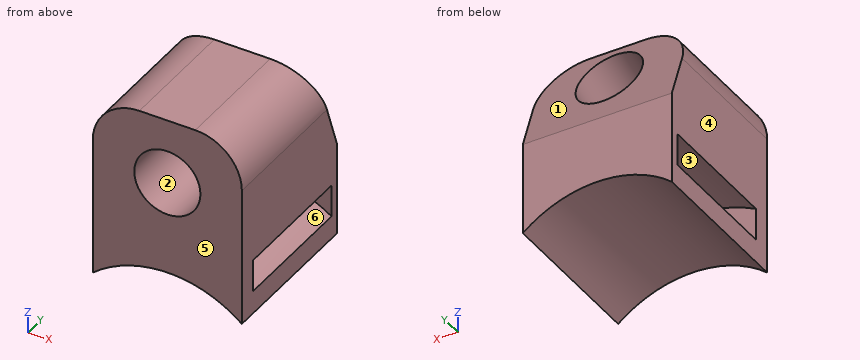
```python
from build123d import *

# Parameters (mm, degrees)
F1_DEPTH  = 15
F3_DEPTH  = 2
F5_R      = 3.55
F8_DEPTH  = 25
F11_DEPTH = 1
F12_R     = 5


with BuildPart() as f1:
    # F0 (on Front) → F1 (new body)
    with BuildSketch(Plane.XZ):
        with BuildLine():
            ThreePointArc((-8, 9.6046863561), (0, 12.5), (8, 9.6046863561))
            Line((8, 9.6046863561), (8, 12.0933866224))
            ThreePointArc((8, 12.0933866224), (0, 14.5), (-8, 12.0933866224))
            Line((-8, 12.0933866224), (-8, 9.6046863561))
        make_face()
    extrude(amount=F1_DEPTH)


with BuildPart() as f1b:
    # F0 (on Front) → F1, piece 2 (new body)
    with BuildSketch(Plane.XZ):
        with BuildLine():
            ThreePointArc((-8, 15.5643824163), (0, 17.5), (8, 15.5643824163))
            Line((8, 15.5643824163), (8, 29.5643824163))
            Line((8, 29.5643824163), (-8, 29.5643824163))
            Line((-8, 29.5643824163), (-8, 15.5643824163))
        make_face()
    extrude(amount=F1_DEPTH)


with BuildPart() as f3:
    # F2 (on face) → F3 (new body)
    with BuildSketch(Plane.XZ.offset(15)):
        with BuildLine():
            ThreePointArc((-8, 9.6046863561), (0, 12.5), (8, 9.6046863561))
            Line((8, 9.6046863561), (8, 12.0933866224))
            ThreePointArc((8, 12.0933866224), (0, 14.5), (-8, 12.0933866224))
            Line((-8, 12.0933866224), (-8, 9.6046863561))
        make_face()
        with BuildLine():
            ThreePointArc((-8, 12.0933866224), (0, 14.5), (8, 12.0933866224))
            Line((8, 12.0933866224), (8, 15.5643824163))
            ThreePointArc((8, 15.5643824163), (0, 17.5), (-8, 15.5643824163))
            Line((-8, 15.5643824163), (-8, 12.0933866224))
        make_face()
        with BuildLine():
            ThreePointArc((-8, 15.5643824163), (0, 17.5), (8, 15.5643824163))
            Line((8, 15.5643824163), (8, 29.5643824163))
            Line((8, 29.5643824163), (-8, 29.5643824163))
            Line((-8, 29.5643824163), (-8, 15.5643824163))
        make_face()
    extrude(amount=F3_DEPTH)


with BuildPart() as f6_tool:
    # F6: sweep along a path in F4
    with BuildLine(Plane.YZ.offset(8)) as f6_path:
        Line((-16, 22.5643824163), (-10, 22.5643824163))
        Line((-10, 22.5643824163), (0, 26.2040847589))
        Line((0, 26.2040847589), (4.1724268391, 27.722723933))
    # F5 (on face) → F6 (sweep)
    with BuildSketch(Plane.XZ.offset(17)):
        with Locations((0, 22.5643824163)):
            Circle(F5_R)
    sweep(path=f6_path.line, transition=Transition.RIGHT)


with BuildPart() as f1b_1:
    add(f1b.part)

    # F6: cut by f6_tool
    add(f6_tool.part, mode=Mode.SUBTRACT)

    # F7 (on face) → F8 (cut)
    with BuildSketch(Plane.YZ.offset(8)):
        Polygon((-3.6397023427, 29.5643824163), (0, 19.5643824163), (0, 29.5643824163), align=None)
    extrude(amount=-F8_DEPTH, mode=Mode.SUBTRACT)


with BuildPart() as f3_1:
    add(f3.part)

    # F6: cut by f6_tool
    add(f6_tool.part, mode=Mode.SUBTRACT)


with BuildPart() as f1_1:
    add(f1.part)

    # F9: union F1b, F3
    add(f1b_1.part)
    add(f3_1.part)

    # F10 (on face) → F11 (join)
    with BuildSketch(Plane(origin=(0, 0, 0), x_dir=(-1, 0, 0), z_dir=(0, 1, 0))):
        with BuildLine():
            ThreePointArc((8, 12.0933866224), (0, 14.5), (-8, 12.0933866224))
            Line((-8, 12.0933866224), (-8, 9.6046863561))
            ThreePointArc((-8, 9.6046863561), (0, 12.5), (8, 9.6046863561))
            Line((8, 9.6046863561), (8, 12.0933866224))
        make_face()
        with BuildLine():
            Line((-8, 15.5643824163), (-8, 12.0933866224))
            ThreePointArc((-8, 12.0933866224), (0, 14.5), (8, 12.0933866224))
            Line((8, 12.0933866224), (8, 15.5643824163))
            ThreePointArc((8, 15.5643824163), (0, 17.5), (-8, 15.5643824163))
        make_face()
        with BuildLine():
            Line((-8, 19.5643824163), (-8, 15.5643824163))
            ThreePointArc((-8, 15.5643824163), (0, 17.5), (8, 15.5643824163))
            Line((8, 15.5643824163), (8, 19.5643824163))
            Line((8, 19.5643824163), (-8, 19.5643824163))
        make_face()
    extrude(amount=-F11_DEPTH)

    # F12
    f12_edges = [f1_1.edges().sort_by_distance(p)[0] for p in [
        (8, -10.319851, 29.564382),
        (-8, -10.319851, 29.564382),
    ]]
    fillet(f12_edges, radius=F12_R)


solid = f1_1.part
```
Part model, mm, in its own coordinate system. Face numbers are marked on the shaded views. A direction names the side the tool comes from. Round coordinates to 2 decimals unless told otherwise and drop trailing zeros. Loops run counter-clockwise (first coordinate to the right, second up) from the corner with the lowest first, then second, coordinate; pieces in that order, holes last. Notation, with made-up numbers: (-7.75, 68.25) -> (5.25, 68.25) arc R17 ccw to (5.25, 100.25) -> close; hole circle Ø5 at (3, 11). An arc over 180 degrees is marked (long way). Use a Markdown table: item, result.
1) Cut at A-A, the plane x = 0. List the corners of the cut face in (y, z), and give its area (3 significant figures).
The answers:
| item | result |
|---|---|
| outline | (-17, 12.5) -> (0, 12.5) -> (0, 19.56) -> (-0.92, 22.09) -> (-9.37, 19.01) -> (-17, 19.01) -> close; (-17, 26.11) -> (-10.63, 26.11) -> (-3.35, 28.76) -> (-3.64, 29.56) -> (-17, 29.56) -> close; hole (-15, 14.5) -> (-1, 14.5) -> (-1, 17.5) -> (-15, 17.5) -> close |
| area | 121 mm2 |
2) Drop a flat-ended pin along its axis: pin 1 Ø3 at (x, y) = (0, -3.5) entering from -Z. Give the stop position or say it passes through.
The answers:
| item | result |
|---|---|
| pin 1 | stops at z = 12.41 |
3) Pull direction Y, two halves, no side cores. Call the marked faces 4, 5 and 6: pulls with the +Y half, pulls with the -Y half, needs draft (parallel to the pull), parting line crosses it, or undercut.
The answers:
| item | result |
|---|---|
| face 4 | needs draft |
| face 5 | pulls with the -Y half |
| face 6 | undercut |
4) Tool access for the marked faces 1, 2 and 3: list every direction of +Z, -Z, +X, -X, +Y, -Y with a clear straight run to the whole face (end or side of a thin tool).
The answers:
| item | result |
|---|---|
| face 1 | +Z, +X, -X, +Y |
| face 2 | -Y |
| face 3 | none |
5) Probe line 1 (Z direction, x = 0, y = -14); line 2 (Y direction, x = 6.25, z = 14.5); line 3 (Z direction, x = 0, y = -15.25). List the from-to ranges inside material, lowest first. Write a range as [from, to].
The answers:
| item | result |
|---|---|
| line 1 | z = [12.5, 14.5], [17.5, 19.01], [26.11, 29.56] |
| line 2 | y = [-17, -15], [-1, 0] |
| line 3 | z = [12.5, 19.01], [26.11, 29.56] |
6) Cut at C-C, the plane z = 12.75. List the corners of the cut face in (x, y).
The answers:
| item | result |
|---|---|
| outline | (-8, -17) -> (8, -17) -> (8, -15) -> (6.91, -15) -> (6.91, -1) -> (8, -1) -> (8, 0) -> (-8, 0) -> (-8, -1) -> (-6.91, -1) -> (-6.91, -15) -> (-8, -15) -> close |
7) Cut at D-D, the plane x = 2.25. List the corners of the cut face in (y, z).
The answers:
| item | result |
|---|---|
| outline | (-17, 12.3) -> (0, 12.3) -> (0, 19.56) -> (-1.19, 22.85) -> (-9.52, 19.82) -> (-17, 19.82) -> close; (-17, 25.31) -> (-10.48, 25.31) -> (-3.07, 28.01) -> (-3.64, 29.56) -> (-17, 29.56) -> close; hole (-15, 14.32) -> (-1, 14.32) -> (-1, 17.35) -> (-15, 17.35) -> close |
8) Cut at B-B, the plane x = 7.25. List the corners of the cut face in (y, z), and give its area (3 significant figures).
The answers:
| item | result |
|---|---|
| outline | (-17, 10.18) -> (0, 10.18) -> (0, 19.56) -> (-2.78, 27.2) -> (-17, 27.2) -> close; hole (-15, 12.56) -> (-1, 12.56) -> (-1, 15.93) -> (-15, 15.93) -> close |
| area | 231 mm2 |
